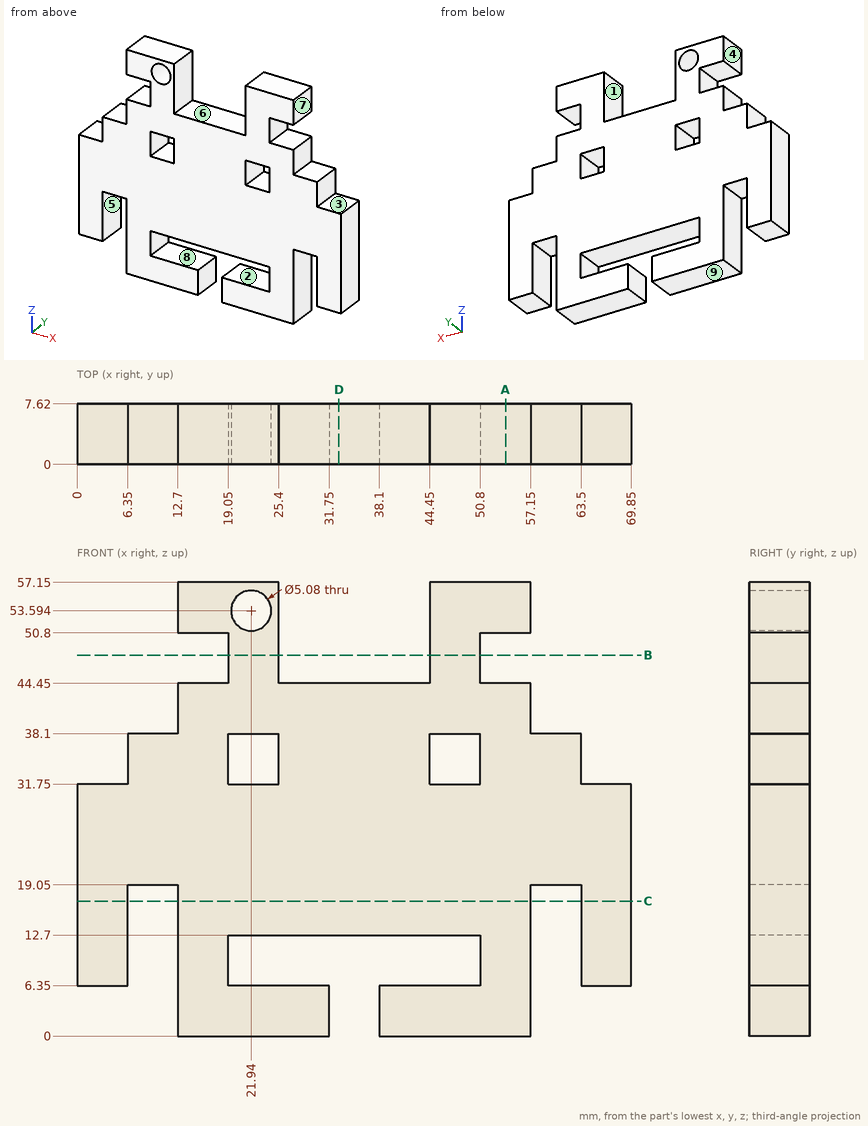
Source: three-view drawing plus pictorial views. Frame: mm from the lowest corner of the part. A direction names the side the tool comes from. Round coordinates to 2 decimals unless told otherwise and drop trailing zeros. Loops run counter-clockwise (first coordinate to the right, second up) from the corner with the lowest first, then second, coordinate; pieces in that order, holes last.
1. Section query D-D on x = 33. Output: boundary loops of the cut face in (y, z), and give its area (3 significant figures).
2. Ray query, L1, parallel to Z at x = 48, y = 5.5; L2, parallel to X at y = 0.5, z = 35; L3, parallel to X at y = 6.5, z = 15.5. Return the intervals inside material, ascending.
3. Section query C-C on z = 17. Output: boundary loops of the cut face in (x, y).
4. Contact query for flat-ended pins moving along their axis: pin 1 (1.9 mm diameter, centred on y = 2, z = 4, fed in from +X); pin 2 (3 mm diameter, centred on x = 21.94, z = 53.59, fed in from +Y); pin 3 (1.9 mm diameter, centred on x = 16.5, y = 3.5, fed in from -Z); pin 4 (1.9 mm diameter, centred on y = 2, z = 34.5, fed in from -X). Output: stop coordinate, or through.
5. Access query for the marked faces 1, 2, 3, 4 and 5. Directions: +Z, -Z, +X, -X, +Y, -Y. A direction counts if a zero-diameter tool reaches every point of the face in a straight line with its end or side. Return the directions, or none.
6. Section query B-B on z = 48. Output: boundary loops of the cut face in (x, y).
7. Mould query, pull axis X, two halves, no side actions, for the marked faces 6, 7, 8 and 9. Classes: released by +X, released by -X, zero draft, split by the parting line, or undercut.
8. Section query A-A on x = 54. Output: boundary loops of the cut face in (y, z), and give its area (3 significant figures).
Answers below:
1. outline: (0, 12.7) - (7.62, 12.7) - (7.62, 44.45) - (0, 44.45) - close
1. area: 242 mm2
2. L1: z = 0 to 6.35, 12.7 to 31.75, 38.1 to 57.15
2. L2: x = 6.35 to 19.05, 25.4 to 44.45, 50.8 to 63.5
2. L3: x = 0 to 6.35, 12.7 to 57.15, 63.5 to 69.85
3. outline: (0, 0) - (6.35, 0) - (6.35, 7.62) - (0, 7.62) - close; (12.7, 0) - (57.15, 0) - (57.15, 7.62) - (12.7, 7.62) - close; (63.5, 0) - (69.85, 0) - (69.85, 7.62) - (63.5, 7.62) - close
4. pin 1: stops at x = 57.15
4. pin 2: passes through
4. pin 3: stops at z = 0
4. pin 4: stops at x = 6.35
5. face 1: +Z, +Y, -Y
5. face 2: +Y, -Y
5. face 3: +Z, +X, +Y, -Y
5. face 4: +Z, -X, +Y, -Y
5. face 5: -Z, +Y, -Y
6. outline: (19.05, 0) - (25.4, 0) - (25.4, 7.62) - (19.05, 7.62) - close; (44.45, 0) - (50.8, 0) - (50.8, 7.62) - (44.45, 7.62) - close
7. face 6: undercut
7. face 7: released by +X
7. face 8: undercut
7. face 9: zero draft
8. outline: (0, 0) - (7.62, 0) - (7.62, 44.45) - (0, 44.45) - close; (0, 50.8) - (7.62, 50.8) - (7.62, 57.15) - (0, 57.15) - close
8. area: 387 mm2
